```python
from build123d import *

# Parameters (mm, degrees)
F0_W     = 16.0737466067
F0_H     = 3.1658632215
F1_DEPTH = 16
F2_R     = 2.3801305446
F2_R_2   = 2.3799092656
F2_R_3   = 2.3780181716
F2_R_4   = 2.3779678295
F3_DEPTH = 1
F5_DEPTH = 5
F6_R     = 1.7583787775
F7_DEPTH = 5


with BuildPart() as f1:
    # F0 (on Front) → F1 (new body)
    with BuildSketch(Plane.XZ):
        with Locations((8.0368733034, 1.5829316108)):
            Rectangle(F0_W, F0_H)
    extrude(amount=F1_DEPTH)

    # F2 (on face) → F3 (join)
    with BuildSketch(Plane.XY.offset(3.1658632215)):
        with Locations((3.9132172242, -11.7802852765)):
            Circle(F2_R)
        with Locations((11.9156921282, -11.7802852765)):
            Circle(F2_R_2)
        with Locations((11.9156921282, -4.0964945219)):
            Circle(F2_R_3)
        with Locations((3.9132172242, -4.0964945219)):
            Circle(F2_R_4)
    extrude(amount=F3_DEPTH)

    # F4 (on face) → F5 (join)
    with BuildSketch(Plane.YZ.offset(16.0737466067)):
        with BuildLine():
            ThreePointArc((-6.5959664397, 0), (-6.3346840784, 0.4988617172), (-6.2445068398, 1.0547389975))
            ThreePointArc((-6.2445068398, 1.0547389975), (-8.5587628976, 2.7229405364), (-9.409804795, 0))
            ThreePointArc((-9.409804795, 0), (-8.0028856173, -0.70363978), (-6.5959664397, 0))
        make_face()
    extrude(amount=F5_DEPTH)

    # F6 (on Right) → F7 (join)
    with BuildSketch(Plane.YZ):
        with Locations((-8.1170331687, 1.0434978176)):
            Circle(F6_R)
    extrude(amount=-F7_DEPTH)


solid = f1.part
```
Geometry check sheet. Reference: the model listing, model coordinates, mm. A direction names the side the tool comes from. Give positions to 0.01 mm unless a question says otherwise; leave off trailing zeros. Loops run counter-clockwise (first coordinate to the right, second up) from the corner with the lowest first, then second, coordinate; pieces in that order, holes last. Notation, with made-up numbers: M -12,-6.5 L 11,-6.5 A13 ccw 11,16.5 Z; hole C -0.75,3.25 d2. An arc over 180 degrees is marked long. Write item = value, one per line. Start each with the question number.
1. Go/stop test with flat-tipped pins: P1, Ø1.5, axis at y = -4.5, z = 2.5, coming from the +X side; P2, Ø4, axis at x = 3.5, y = -13, coming from the -Z side; P3, Ø1.5, axis at x = 14, z = 1.5, coming from the +Y side. Record where each tip stops, or that it passes through.
2. Tool access check on faces 4 (the face through (4, -4, 4.166)), 5 (the face through (9.54, -3.99, 3.66)). Record the directions out of +Z, -Z, +X, -X, +Y, -Y that give a thin tool (end or side, any length) a straight path to the whole face; none if there is none.
3. Section check B-B, the plane z = 0.6. Enter the section's corners in (x, y).
4. Draft check along X on faces 1 (the face through (-5, -8, 1)), 2 (the face through (5.011, -6.206, 3.659)), 3 (the face through (-2.46, -6.44, 1.57)). Enter one of: +X half, -X half, draft (parallel to the pull), parting line (faces both ways), or undercut.
5. Thickness scan on probe 1 along Z at (x, y) = (9.75, -11.25); probe 2 along X at (y, z) = (-8, 2.85); probe 3 along Z at (x, y) = (15.5, -8). Record the ranges inside material, lowest first.
6. Section check C-C, the plane z = 3.6. Enter the section's corners in (x, y), plus the area to 3 significant figures.
7. Section check A-A, the plane y = -2. Enter the section's corners in (x, z), plus the area to 3 significant figures.
Values follow:
q1.P1 = 16.07
q1.P2 = 0
q1.P3 = 0
q2.face_4 = +Z, +X, -X, +Y, -Y
q2.face_5 = +Z
q3.outline = M -5,-9.82 L 0,-9.82 L 0,-16 L 16.07,-16 L 16.07,-9.7 L 21.07,-9.7 L 21.07,-6.3 L 16.07,-6.3 L 16.07,0 L 0,0 L 0,-6.42 L -5,-6.42 Z
q4.face_1 = -X half
q4.face_2 = undercut
q4.face_3 = draft
q5.probe_1 = 0 to 4.17
q5.probe_2 = 0 to 16.07
q5.probe_3 = 0 to 3.17
q6.outline = C 3.91,-11.78 d4.76; C 3.91,-4.1 d4.76; C 11.92,-11.78 d4.76; C 11.92,-4.1 d4.76
q6.area = 71.1 mm^2
q7.outline = M 0,0 L 16.07,0 L 16.07,3.17 L 13.04,3.17 L 13.04,4.17 L 10.79,4.17 L 10.79,3.17 L 5.04,3.17 L 5.04,4.17 L 2.79,4.17 L 2.79,3.17 L 0,3.17 Z
q7.area = 55.4 mm^2
